from build123d import *

# Parameters (mm, degrees)
CROQUIS1_R                 = 12.5
SALIENTE_EXTRUIR1_DEPTH    = 15
CROQUIS2_W                 = 23.106060606
CROQUIS2_H                 = 20
CROQUIS2_H_2               = 22
CORTAR_EXTRUIR1_DEPTH      = 26
CORTAR_EXTRUIR1_DEPTH_BACK = 26
CROQUIS3_R                 = 10
CORTAR_EXTRUIR2_DEPTH      = 16
CORTAR_EXTRUIR2_DEPTH_BACK = 16


with BuildPart() as part:
    # Croquis1 → Saliente-Extruir1 (new body, symmetric)
    with BuildSketch(Plane(origin=(0, 0, 0), x_dir=(1, 0, 0), z_dir=(0, 1, 0))):
        with BuildLine():
            Line((-165.946969697, 12.464078321), (-1.893939394, 24.928156642))
            ThreePointArc((-1.893939394, 24.928156642), (0, 25), (1.893939394, 24.928156642))
            Line((1.893939394, 24.928156642), (165.946969697, 12.464078321))
            ThreePointArc((165.946969697, 12.464078321), (177.5, 0), (165.946969697, -12.464078321))
            Line((165.946969697, -12.464078321), (1.893939394, -24.928156642))
            ThreePointArc((1.893939394, -24.928156642), (0, -25), (-1.893939394, -24.928156642))
            Line((-1.893939394, -24.928156642), (-165.946969697, -12.464078321))
            ThreePointArc((-165.946969697, -12.464078321), (-177.5, 0), (-165.946969697, 12.464078321))
        make_face()
        Circle(CROQUIS1_R, mode=Mode.SUBTRACT)
    extrude(amount=SALIENTE_EXTRUIR1_DEPTH, both=True)

    # Croquis2 → Cortar-Extruir1 (cut, two sides)
    with BuildSketch(Plane.XY) as cortar_extruir1_sk:
        with Locations((165.946969697, 0)):
            Rectangle(CROQUIS2_W, CROQUIS2_H)
        with Locations((-165.946969697, 0)):
            Rectangle(CROQUIS2_W, CROQUIS2_H_2)
    extrude(amount=CORTAR_EXTRUIR1_DEPTH, mode=Mode.SUBTRACT)
    extrude(cortar_extruir1_sk.sketch, amount=-CORTAR_EXTRUIR1_DEPTH_BACK, mode=Mode.SUBTRACT)

    # Croquis3 → Cortar-Extruir2 (cut, two sides)
    with BuildSketch(Plane(origin=(0, 0, 0), x_dir=(1, 0, 0), z_dir=(0, 1, 0))) as cortar_extruir2_sk:
        with Locations((-165, 0)):
            Circle(CROQUIS3_R)
        with Locations((165, 0)):
            Circle(CROQUIS3_R)
    extrude(amount=CORTAR_EXTRUIR2_DEPTH, mode=Mode.SUBTRACT)
    extrude(cortar_extruir2_sk.sketch, amount=-CORTAR_EXTRUIR2_DEPTH_BACK, mode=Mode.SUBTRACT)


solid = part.part
The listing builds one solid part. Answer for the finished solid, in the listing's coordinates (mm). A direction names the side the tool comes from. Round coordinates to 2 decimals unless told otherwise and drop trailing zeros. Loops run counter-clockwise (first coordinate to the right, second up) from the corner with the lowest first, then second, coordinate; pieces in that order, holes last. Notation, with made-up numbers: M -14.75,40.25 L 3.25,40.25 A19 cw 3.25,53.25 Z; hole C 59,-11 d6. An arc over 180 degrees is marked long. Return JSON: item names as keys, results as strings.
Q1. Find the intervals of material crossed by line 1 along Z through (x, y) = (-165, 12.3); line 2 along X through (y, z) = (-13.25, 4.5); line 3 along X through (y, z) = (10.25, -1.5), in increasing order. Write a range as from..to.
Results list:
{"line 1": "z = -12.54..-10, 10..12.54", "line 2": "x = -176.66..-173.93, -156.07..-11.66, 11.66..156.07, 173.93..176.66", "line 3": "x = -154.39..-12.41, 12.41..155.11, 174.89..177.41"}
Q2. Find section C-C, the plane x = 38.5. Determine the outline of the cut face in (y, z).
Results list:
{"outline": "M -15,-22.15 L 15,-22.15 L 15,22.15 L -15,22.15 Z"}
Q3. Which of the six approach directions +Z, -Z, +X, -X, +Y, -Y give full straight-line access (tool end or side, diameter ignored) to faces 1 (the face through (154.8, 10, 0.1)), 2 (the face through (-82.772, 0.21, 18.783)), 3 (the face through (-154.88, 11, -0.93))?
Results list:
{"face 1": "+Z, -Z, +X", "face 2": "+Z, -X, +Y, -Y", "face 3": "+Z, -Z, -X"}
Q4. Find section B-B, the plane y = -4.25. Determine the outline of the cut face in (x, z).
Results list:
{"outline": "M -154.39,-13.34 L -1.89,-24.93 A25 ccw 1.89,-24.93 L 154.39,-13.34 L 154.39,13.34 L 1.89,24.93 A25 ccw -1.89,24.93 L -154.39,13.34 Z; hole C 0,0 d25"}
Q5. Each of these flat-tipped pins is pushed along its axis until it touches: pin 1 Ø6 at (x, y) = (-92, 8.5) entering from +Z; pin 2 Ø2 at (x, y) = (-63, 1) entering from -Z; pin 3 Ø10 at (y, z) = (-2, 5.5) entering from +X; pin 4 Ø16 at (x, z) = (165, 0) entering from +Y. Where does it stop, or does it pass through?
Results list:
{"pin 1": "stops at z = 18.31", "pin 2": "stops at z = -20.36", "pin 3": "stops at x = 154.39", "pin 4": "passes through"}
Q6. Find section D-D, the plane z = 17. Determine the outline of the cut face in (x, y), plus the area to 3 significant figures.
Results list:
{"outline": "M -106.24,-15 L 106.24,-15 L 106.24,15 L -106.24,15 Z", "area": "6,370 mm2"}
Q7. The mould has two halves that part along Z. Classify faces 4 (the face through (-154.88, -11, -0.93)), 5 (the face through (-177.497, -12.972, 0.262)), 6 (the face through (-155.763, -12.972, 3.83)): released by +Z, released by -Z, zero draft, split by the parting line, or undercut.
Results list:
{"face 4": "zero draft", "face 5": "split by the parting line", "face 6": "undercut"}
Q8. Find section A-A, the plane z = 0. State how many separate pieces and enclosed holes the cut face has, plus the area to 3 significant figures.
Results list:
{"separate pieces": "6", "enclosed holes": "0", "area": "8,570 mm2"}
